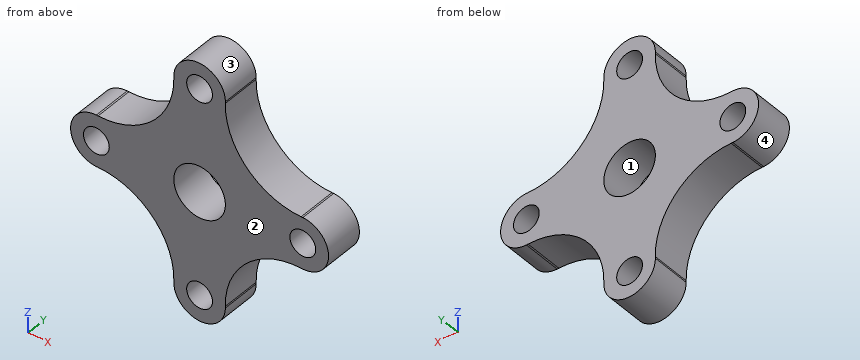
from build123d import *

# Parameters (mm, degrees)
F0_R     = 6.35
F0_R_2   = 12.7
F1_DEPTH = 19.05


with BuildPart() as f1:
    # F0 (on Front) → F1 (new body)
    with BuildSketch(Plane.XZ):
        with BuildLine():
            ThreePointArc((12.7, 50.8), (12.684041, 50.384765), (12.672808, 49.969374))
            ThreePointArc((12.672808, 49.969374), (12.6932, 50.384465), (12.7, 50.8))
        make_face()
        with BuildLine():
            ThreePointArc((49.969374, 12.672808), (23.362469, 23.362469), (12.672808, 49.969374))
            ThreePointArc((12.672808, 49.969374), (12.684041, 50.384765), (12.7, 50.8))
            ThreePointArc((12.7, 50.8), (0, 63.5), (-12.7, 50.8))
            ThreePointArc((-12.7, 50.8), (-12.684041, 50.384765), (-12.672808, 49.969374))
            ThreePointArc((-12.672808, 49.969374), (-23.362469, 23.362469), (-49.969374, 12.672808))
            ThreePointArc((-49.969374, 12.672808), (-50.384765, 12.684041), (-50.8, 12.7))
            ThreePointArc((-50.8, 12.7), (-63.5, 0), (-50.8, -12.7))
            ThreePointArc((-50.8, -12.7), (-50.384765, -12.684041), (-49.969374, -12.672808))
            ThreePointArc((-49.969374, -12.672808), (-23.362469, -23.362469), (-12.672808, -49.969374))
            ThreePointArc((-12.672808, -49.969374), (-12.684041, -50.384765), (-12.7, -50.8))
            ThreePointArc((-12.7, -50.8), (0, -63.5), (12.7, -50.8))
            ThreePointArc((12.7, -50.8), (12.684041, -50.384765), (12.672808, -49.969374))
            ThreePointArc((12.672808, -49.969374), (23.362469, -23.362469), (49.969374, -12.672808))
            ThreePointArc((49.969374, -12.672808), (50.384765, -12.684041), (50.8, -12.7))
            ThreePointArc((50.8, -12.7), (63.5, 0), (50.8, 12.7))
            ThreePointArc((50.8, 12.7), (50.384765, 12.684041), (49.969374, 12.672808))
        make_face()
        with Locations((0, -50.8)):
            Circle(F0_R, mode=Mode.SUBTRACT)
        with Locations((-50.8, 0)):
            Circle(F0_R, mode=Mode.SUBTRACT)
        Circle(F0_R_2, mode=Mode.SUBTRACT)
        with Locations((50.8, 0)):
            Circle(F0_R, mode=Mode.SUBTRACT)
        with Locations((0, 50.8)):
            Circle(F0_R, mode=Mode.SUBTRACT)
        with BuildLine():
            ThreePointArc((50.8, 12.7), (50.384465, 12.6932), (49.969374, 12.672808))
            ThreePointArc((49.969374, 12.672808), (50.384765, 12.684041), (50.8, 12.7))
        make_face()
        with BuildLine():
            ThreePointArc((-12.672808, 49.969374), (-12.684041, 50.384765), (-12.7, 50.8))
            ThreePointArc((-12.7, 50.8), (-12.6932, 50.384465), (-12.672808, 49.969374))
        make_face()
        with BuildLine():
            ThreePointArc((49.969374, -12.672808), (50.384465, -12.6932), (50.8, -12.7))
            ThreePointArc((50.8, -12.7), (50.384765, -12.684041), (49.969374, -12.672808))
        make_face()
        with BuildLine():
            ThreePointArc((-50.8, 12.7), (-50.384765, 12.684041), (-49.969374, 12.672808))
            ThreePointArc((-49.969374, 12.672808), (-50.384465, 12.6932), (-50.8, 12.7))
        make_face()
        with BuildLine():
            ThreePointArc((12.7, -50.8), (12.6932, -50.384465), (12.672808, -49.969374))
            ThreePointArc((12.672808, -49.969374), (12.684041, -50.384765), (12.7, -50.8))
        make_face()
        with BuildLine():
            ThreePointArc((-49.969374, -12.672808), (-50.384765, -12.684041), (-50.8, -12.7))
            ThreePointArc((-50.8, -12.7), (-50.384465, -12.6932), (-49.969374, -12.672808))
        make_face()
        with BuildLine():
            ThreePointArc((-12.672808, -49.969374), (-12.6932, -50.384465), (-12.7, -50.8))
            ThreePointArc((-12.7, -50.8), (-12.684041, -50.384765), (-12.672808, -49.969374))
        make_face()
    extrude(amount=F1_DEPTH)


solid = f1.part
Read the model definition and answer for the solid it produces. Units are mm, in the model's axes. Face numbers are marked on the shaded views. Coordinates: 2 decimals unless noted, no trailing zeros. Loops run counter-clockwise (first coordinate to the right, second up) from the corner with the lowest first, then second, coordinate; pieces in that order, holes last. Notation, with made-up numbers: (-10, 71.5) - (39, 71.5) arc R20 ccw to (39, 99.5) - close; hole circle Ø10 at (4, -6.5). An arc over 180 degrees is marked (long way). Answer in a Markdown table with one row per item.
Q1. Find section A-A on x = 0. Write down the section's boundary in (y, z), plus the area to 3 significant figures.
Here are the results:
| item | result |
|---|---|
| outline | (-19.05, -63.5) - (0, -63.5) - (0, -57.15) - (-19.05, -57.15) - close; (-19.05, -44.45) - (0, -44.45) - (0, -12.7) - (-19.05, -12.7) - close; (-19.05, 12.7) - (0, 12.7) - (0, 44.45) - (-19.05, 44.45) - close; (-19.05, 57.15) - (0, 57.15) - (0, 63.5) - (-19.05, 63.5) - close |
| area | 1,450 mm^2 |
Q2. Find section D-D on x = -46.5. Write down the section's boundary in (y, z).
Here are the results:
| item | result |
|---|---|
| outline | (-19.05, -12.76) - (0, -12.76) - (0, -4.67) - (-19.05, -4.67) - close; (-19.05, 4.67) - (0, 4.67) - (0, 12.76) - (-19.05, 12.76) - close |
Q3. Find section B-B on z = 0. Write down the section's boundary in (x, y).
Here are the results:
| item | result |
|---|---|
| outline | (-63.5, -19.05) - (-57.15, -19.05) - (-57.15, 0) - (-63.5, 0) - close; (-44.45, -19.05) - (-12.7, -19.05) - (-12.7, 0) - (-44.45, 0) - close; (12.7, -19.05) - (44.45, -19.05) - (44.45, 0) - (12.7, 0) - close; (57.15, -19.05) - (63.5, -19.05) - (63.5, 0) - (57.15, 0) - close |
Q4. The mould has two halves that part along Z. Classify the marked faces 1, 2, 3 and 4: pulls with the +Z half, pulls with the -Z half, needs draft (parallel to the pull), parting line crosses it, or undercut.
Here are the results:
| item | result |
|---|---|
| face 1 | undercut |
| face 2 | needs draft |
| face 3 | pulls with the +Z half |
| face 4 | parting line crosses it |
Q5. Given P1, Ø6, axis at y = -5.5, z = 8, coming from the -X side; P2, Ø1.5, axis at y = -15, z = -46, coming from the +X side; P3, Ø2, axis at y = -12.5, z = -41.5, coming from the +X side, each flat-ended and moving along its own axis, determine where each tip first touches the part or whether it passes through.
Here are the results:
| item | result |
|---|---|
| P1 | stops at x = -62.47 |
| P2 | stops at x = 12.88 |
| P3 | stops at x = 13.71 |
Q6. Straight lines are drawn through the part: line 1 along Z through (x, y) = (0, -12.5); line 2 along Z through (x, y) = (50.8, -9); line 3 along X through (y, z) = (-6.25, -4.5). For each, find the intervals that lie inside material, in ascending order. Write a range as [from, to].
Here are the results:
| item | result |
|---|---|
| line 1 | z = [-63.5, -57.15], [-44.45, -12.7], [12.7, 44.45], [57.15, 63.5] |
| line 2 | z = [-12.7, -6.35], [6.35, 12.7] |
| line 3 | x = [-62.68, -55.28], [-46.32, -11.88], [11.88, 46.32], [55.28, 62.68] |
Q7. Find section C-C on y = -5.75. Write down the section's boundary in (x, z).
Here are the results:
| item | result |
|---|---|
| outline | (-50.8, -12.7) arc R12.7 ccw to (-49.97, -12.67) arc R36.53 cw to (-12.67, -49.97) arc R12.7 ccw to (-12.7, -50.8) arc R12.7 ccw to (12.7, -50.8) arc R12.7 ccw to (12.67, -49.97) arc R36.53 cw to (49.97, -12.67) arc R12.7 ccw to (50.8, -12.7) arc R12.7 ccw to (50.8, 12.7) arc R12.7 ccw to (49.97, 12.67) arc R36.53 cw to (12.67, 49.97) arc R12.7 ccw to (12.7, 50.8) arc R12.7 ccw to (-12.7, 50.8) arc R12.7 ccw to (-12.67, 49.97) arc R36.53 cw to (-49.97, 12.67) arc R12.7 ccw to (-50.8, 12.7) arc R12.7 ccw to start; hole circle Ø12.7 at (-50.8, 0); hole circle Ø25.4 at (0, 0); hole circle Ø12.7 at (0, -50.8); hole circle Ø12.7 at (0, 50.8); hole circle Ø12.7 at (50.8, 0) |
